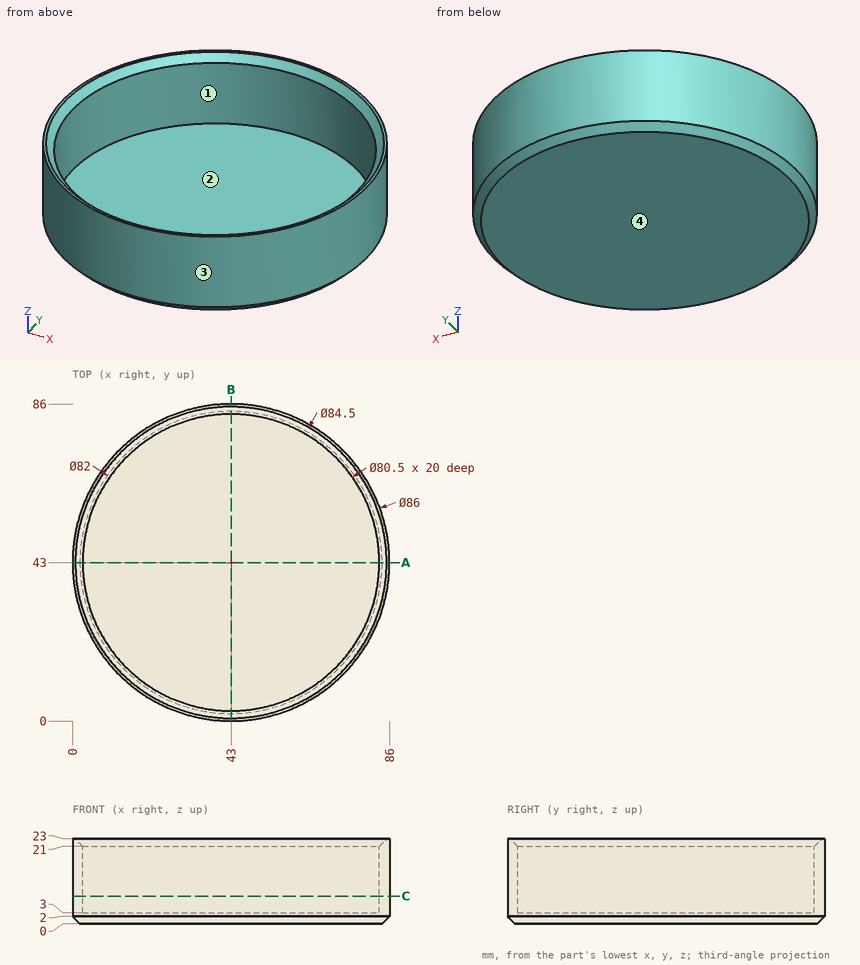
Input: dimensioned drawing with shaded views. Units: mm. Origin: part minimum x, y, z. Coordinates: 2 decimals unless noted, no trailing zeros. Order: outer loops, then holes, each group sorted by start corner. A loop starts at its lowest first (then second) coordinate and runs counter-clockwise, first axis right, second up.
1. Contact query for flat-ended pins moving along their axis: P1, Ø1, axis at y = 23.5, z = 20.5, coming from the +X side; P2, Ø1, axis at x = 35.5, y = 32, coming from the +Z side; P3, Ø12, axis at x = 73.5, z = 12.5, coming from the -Y side; P4, Ø8, axis at x = 75, y = 16, coming from the +Z side. Output: stop coordinate, or through.
Checked values:
P1: stops at x = 81.57
P2: stops at z = 3
P3: stops at y = 7.66
P4: stops at z = 23
2. Cut plane C-C, the plane z = 7.5. Return loops of the section in (x, y), plus the area to 3 significant figures.
Checked values:
outline: circle Ø86 at (43, 43); hole circle Ø80.5 at (43, 43)
area: 719 mm2
3. Ray query, line 1 along Y through (x, z) = (43, 7.5); line 2 along Z through (x, y) = (12.5, 66); line 3 along Y through (x, z) = (61, 10.5). Return the intervals inside material, ascending.
Checked values:
line 1: y = 0 to 2.75, 83.25 to 86
line 2: z = 0 to 3
line 3: y = 3.95 to 7, 79 to 82.05
4. Draft query along X for the marked faces 1, 2, 3 and 4. Return one class per face: +X half, -X half, draft (parallel to the pull), parting line (faces both ways), or undercut.
Checked values:
face 1: undercut
face 2: undercut
face 3: parting line
face 4: draft
5. Cut plane A-A, the plane y = 43. Return loops of the section in (x, z), plus the area to 3 significant figures.
Checked values:
outline: (0, 2) - (2, 0) - (84, 0) - (86, 2) - (86, 23) - (85.25, 23) - (83.25, 21) - (83.25, 3) - (2.75, 3) - (2.75, 21) - (0.75, 23) - (0, 23) - close
area: 360 mm2
